from build123d import *


with BuildPart() as part:
    # Sketch1 → Revolve-Thin3 (revolve)
    with BuildSketch(Plane.XY):
        with BuildLine():
            ThreePointArc((18.551548743, 431.8), (54.132203955, 217.201745506), (66.04, 0))
            Line((66.04, 0), (63.5, 0))
            Line((63.5, 0), (63.5, -127))
            Line((63.5, -127), (60.325, -127))
            Line((60.325, -127), (60.325, 3.175))
            Line((60.325, 3.175), (62.862459123, 3.175))
            ThreePointArc((62.862459123, 3.175), (50.80205754, 218.432575212), (15.452434998, 431.109986233))
            Line((15.452434998, 431.109986233), (18.551548743, 431.8))
        make_face()
    revolve(axis=Axis((0, 0, 0), (0, 1, 0)))


solid = part.part
Check sheet for the modelled part. Datum: model origin and axes. Units: mm. Give positions to 0.01 mm unless a question says otherwise; leave off trailing zeros. One line per item, written item: value. Start each with the question number.
Item 1: Draft check along Z on faces 1 (the cylindrical face through (-60.267, -61.001, -2.652)), 2 (the flat face through (-35, 0, -54)), 3 (the cylindrical face through (-13.77, -64.39, 61.99)), 4 (the flat face through (24, 3.175, -56)). Enter one of: +Z half, -Z half, draft (parallel to the pull), parting line (faces both ways), or undercut.
Item 2: Gauge pin test, flat ends, axial feed: pin 1 (2 mm diameter, centred on y = -33, z = 32.5, fed in from +X); pin 2 (10 mm diameter, centred on y = 346, z = 37, fed in from +X); pin 3 (2 mm diameter, centred on y = 230, z = 12, fed in from +X). Record the tip position at first contact, or that the pin passes through.
Item 3: Material ranges on probe 1 along Z at (x, y) = (0, -36) (3 decimals); probe 2 along Z at (x, y) = (14, 15), recorded low to high. Write a range as from..to.
Results list:
1. face 1: undercut
1. face 2: draft
1. face 3: parting line
1. face 4: undercut
2. pin 1: x = 55.14
2. pin 2: x = 15.98
2. pin 3: x = 51.55
3. probe 1: -63.5..-60.325, 60.325..63.5
3. probe 2: -64.48..-61.23, 61.23..64.48
